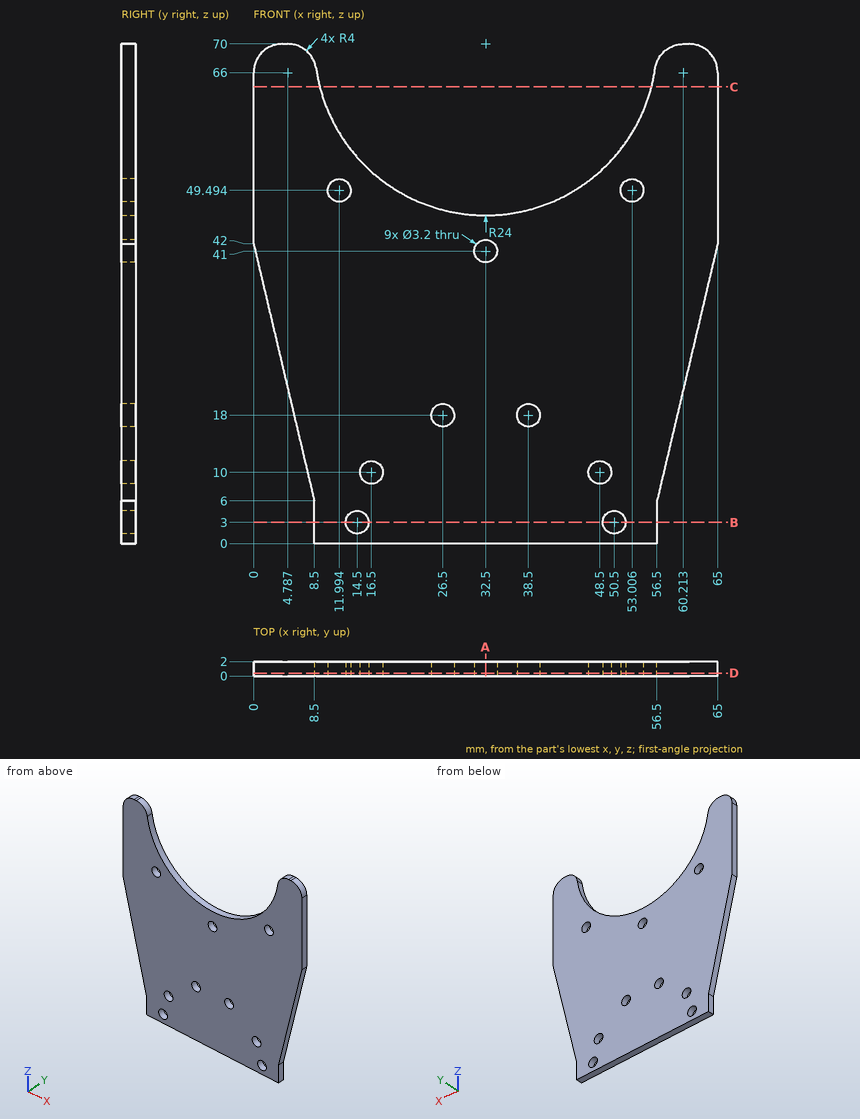
Verification items for this drawing (mm, ordinates from the low corner). Coordinates: 2 decimals unless noted, no trailing zeros. Write each loop counter-clockwise with the first axis right and the second up, starting at its lowest first coordinate (ties: lowest second). Pieces come first, ordered by that corner, then holes. Notation, with made-up numbers: (13.5, 79) -> (23.5, 79) arc R8 ccw to (23.5, 89) -> close; hole circle Ø4 at (72.5, 41.5). An arc over 180 degrees is marked (long way). One line per item, written item: value. Start each with the question number.
Q1. Cross-section at A-A on x = 32.5. Enter the section's corners in (y, z).
Q2. Cross-section at B-B on z = 3. Enter the section's corners in (x, y).
Q3. Thickness scan on L1, parallel to X at y = 0.8, z = 9; L2, parallel to X at y = 1.2, z = 18; L3, parallel to Z at x = 54, y = 0.6 (1 decimal). Record the ranges inside material, lowest first. Write a range as from..to.
Q4. Cross-section at C-C on z = 64. Enter the section's corners in (x, y).
Q5. Cross-section at D-D on y = 0.4. State how many separate pieces and enclosed holes the cut face has, and give its area (3 significant figures).
Checked values:
1. outline: (0, 0) -> (2, 0) -> (2, 39.4) -> (0, 39.4) -> close; (0, 42.6) -> (2, 42.6) -> (2, 46) -> (0, 46) -> close
2. outline: (8.5, 0) -> (12.9, 0) -> (12.9, 2) -> (8.5, 2) -> close; (16.1, 0) -> (48.9, 0) -> (48.9, 2) -> (16.1, 2) -> close; (52.1, 0) -> (56.5, 0) -> (56.5, 2) -> (52.1, 2) -> close
3. L1: x = 7.79..15.25, 17.75..47.25, 49.75..57.21
3. L2: x = 5.67..24.9, 28.1..36.9, 40.1..59.33
3. L3: z = 0..48.2, 50.7..59.3
4. outline: (0, 0) -> (9.26, 0) -> (9.26, 2) -> (0, 2) -> close; (55.74, 0) -> (65, 0) -> (65, 2) -> (55.74, 2) -> close
5. separate pieces: 1
5. enclosed holes: 9
5. area: 3,150 mm²
